Read the model definition and answer for the solid it produces. Units are mm, in the model's axes. A direction names the side the tool comes from. Give positions to 0.01 mm unless a question says otherwise; leave off trailing zeros. Write each loop counter-clockwise with the first axis right and the second up, starting at its lowest first coordinate (ties: lowest second). Pieces come first, ordered by that corner, then holes. Notation, with made-up numbers: M 21.25,-30 L 75.25,-30 A15 ccw 75.25,-4 Z; hole C 30.25,45.25 d5. An arc over 180 degrees is marked long. Use a Markdown table: item, result. Add a question column.
Item 1: A cutting plane is placed at B-B on z = 0.15. Count the separate pieces of the cut face and the enclosed holes in it, then the cut area to 3 significant figures.
Item 2: A cutting plane is placed at C-C on x = 12.5. Determine the outline of the cut face in (y, z).
Item 3: A cutting plane is placed at A-A on x = -25.4. Determine the outline of the cut face in (y, z), then the cut area to 3 significant figures.
Item 4: For faces 1 (the cylindrical face through (6.8, -11.5, 0)), 2 (the flat face through (69.85, 0, 0)), determine the directions among +Z, -Z, +X, -X, +Y, -Y from which every point of the face is accessible in a straight line to the end or side of a thin tool.
Item 5: Consider probe 1 along Y at (x, z) = (4, 0.3); probe 2 along Y at (x, z) = (63.5, 0.7) (3 decimals); probe 3 along X at (y, z) = (4.5, -0.1). Determine where each line is inside the solid, lowest interval first. Write a range as [from, to].
from build123d import *

# Parameters (mm, degrees)
SKETCH1_W           = 139.7
SKETCH1_H           = 50.8
SKETCH1_R           = 3.175
SKETCH1_R_2         = 14.2875
BOSS_EXTRUDE1_DEPTH = 1.143
FILLET1_R           = 6.35
CUT_EXTRUDE1_DEPTH  = 2.54
FILLET2_R           = 2.54


with BuildPart() as part:
    # Sketch1 → Boss-Extrude1 (new, symmetric)
    with BuildSketch(Plane.XY):
        Rectangle(SKETCH1_W, SKETCH1_H)
        with Locations((-63.5, 0)):
            Circle(SKETCH1_R, mode=Mode.SUBTRACT)
        with Locations((63.5, 0)):
            Circle(SKETCH1_R, mode=Mode.SUBTRACT)
        with Locations((-25.4, 0)):
            Circle(SKETCH1_R_2, mode=Mode.SUBTRACT)
        with Locations((25.4762, 0)):
            Circle(SKETCH1_R_2, mode=Mode.SUBTRACT)
    extrude(amount=BOSS_EXTRUDE1_DEPTH, both=True)

    # Fillet1
    fillet1_edges = [part.edges().sort_by_distance(p)[0] for p in [
        (69.85, -25.4, 0),
        (-69.85, -25.4, 0),
        (-69.85, 25.4, 0),
        (69.85, 25.4, 0),
    ]]
    fillet(fillet1_edges, radius=FILLET1_R)

    # Sketch2 → Cut-Extrude1 (cut)
    with BuildSketch(Plane.XY.offset(1.143)):
        with BuildLine():
            Line((-57.15, 12.7), (-57.15, -12.7))
            Line((-57.15, -12.7), (-41.667034341, -12.7))
            ThreePointArc((-41.667034341, -12.7), (-46.0375, 0), (-41.667034341, 12.7))
            Line((-41.667034341, 12.7), (-57.15, 12.7))
        make_face()
        with BuildLine():
            ThreePointArc((-4.7625, 0), (-5.885680547, -6.715485278), (-9.132965659, -12.7))
            Line((-9.132965659, -12.7), (9.209165659, -12.7))
            ThreePointArc((9.209165659, -12.7), (4.8387, 0), (9.209165659, 12.7))
            Line((9.209165659, 12.7), (-9.132965659, 12.7))
            ThreePointArc((-9.132965659, 12.7), (-5.885680547, 6.715485278), (-4.7625, 0))
        make_face()
        with BuildLine():
            ThreePointArc((46.1137, 0), (44.990519453, -6.715485278), (41.743234341, -12.7))
            Line((41.743234341, -12.7), (57.15, -12.7))
            Line((57.15, -12.7), (57.15, 12.7))
            Line((57.15, 12.7), (41.743234341, 12.7))
            ThreePointArc((41.743234341, 12.7), (44.990519453, 6.715485278), (46.1137, 0))
        make_face()
    extrude(amount=-CUT_EXTRUDE1_DEPTH, mode=Mode.SUBTRACT)

    # Fillet2
    fillet2_edges = [part.edges().sort_by_distance(p)[0] for p in [
        (-41.667034341, 12.7, 0),
        (-41.667034341, -12.7, 0),
        (-57.15, -12.7, 0),
        (-57.15, 12.7, 0),
        (9.209165659, 12.7, 0),
        (9.209165659, -12.7, 0),
        (-9.132965659, -12.7, 0),
        (-9.132965659, 12.7, 0),
        (41.743234341, -12.7, 0),
        (41.743234341, 12.7, 0),
        (57.15, 12.7, 0),
        (57.15, -12.7, 0),
    ]]
    fillet(fillet2_edges, radius=FILLET2_R)


solid = part.part
Filled in:
| question | item | result |
|---|---|---|
| 1 | separate pieces | 1 |
| 1 | enclosed holes | 7 |
| 1 | area | 4,810 mm² |
| 2 | outline | M -25.4,-1.14 L -5.98,-1.14 L -5.98,1.14 L -25.4,1.14 Z; M 5.98,-1.14 L 25.4,-1.14 L 25.4,1.14 L 5.98,1.14 Z |
| 3 | outline | M -25.4,-1.14 L -14.29,-1.14 L -14.29,1.14 L -25.4,1.14 Z; M 14.29,-1.14 L 25.4,-1.14 L 25.4,1.14 L 14.29,1.14 Z |
| 3 | area | 50.8 mm² |
| 4 | face 1 | +Z, -Z |
| 4 | face 2 | +Z, -Z, +X, +Y, -Y |
| 5 | probe 1 | [-25.4, -12.7], [12.7, 25.4] |
| 5 | probe 2 | [-25.4, -3.175], [3.175, 25.4] |
| 5 | probe 3 | [-69.85, -57.15], [-45.54, -38.96], [-11.84, -5.26], [5.34, 11.92], [39.04, 45.62], [57.15, 69.85] |
